The listing builds one solid part. Answer for the finished solid, in the listing's coordinates (mm). A direction names the side the tool comes from. Give positions to 0.01 mm unless a question says otherwise; leave off trailing zeros. Write each loop counter-clockwise with the first axis right and the second up, starting at its lowest first coordinate (ties: lowest second). Pieces come first, ordered by that corner, then holes. Notation, with made-up numbers: M -1.5,15.5 L 25.5,15.5 A23 ccw 25.5,41.5 Z; hole C 75,60.25 d8. An arc over 180 degrees is marked long. Return JSON: item names as keys, results as strings.
from build123d import *

# Parameters (mm, degrees)
F0_W     = 110
F0_H     = 40
F1_DEPTH = 2
F2_W     = 45
F2_H     = 29
F3_DEPTH = 2.001
F4_R     = 2
F5_R     = 4


with BuildPart() as f1:
    # F0 (on Top) → F1 (new body)
    with BuildSketch(Plane.XY):
        Rectangle(F0_W, F0_H)
    extrude(amount=F1_DEPTH)

    # F2 (on face) → F3 (cut, through all)
    with BuildSketch(Plane.XY.offset(2)):
        Rectangle(F2_W, F2_H)
    extrude(amount=-F3_DEPTH, mode=Mode.SUBTRACT)

    # F4
    f4_edges = [f1.edges().sort_by_distance(p)[0] for p in [
        (-22.5, 14.5, 1),
        (22.5, 14.5, 1),
        (-22.5, -14.5, 1),
        (22.5, -14.5, 1),
    ]]
    fillet(f4_edges, radius=F4_R)

    # F5
    f5_edges = [f1.edges().sort_by_distance(p)[0] for p in [
        (-55, -20, 1),
        (-55, 20, 1),
        (55, 20, 1),
        (55, -20, 1),
    ]]
    fillet(f5_edges, radius=F5_R)


solid = f1.part
Item 1: Determine the mould class of faces 3 (the flat face through (55, 0, 1)), 4 (the cylindrical face through (53.797, -18.859, 1.014)), 5 (the cylindrical face through (-21.9, -13.93, 0.99)) for opening direction Y: +Y half, -Y half, draft (parallel to the pull), parting line (faces both ways), or undercut.
Geometry results:
{"face 3": "draft", "face 4": "-Y half", "face 5": "undercut"}
Item 2: A cutting plane is placed at A-A, the plane y = 9. Write down the section's boundary in (x, z).
Geometry results:
{"outline": "M -55,0 L -22.5,0 L -22.5,2 L -55,2 Z; M 22.5,0 L 55,0 L 55,2 L 22.5,2 Z"}
Item 3: Find the intervals of material crossed by line 1 (Y direction, x = 2.5, z = 0.4); line 2 (X direction, y = -2, z = 1.8); line 3 (X direction, y = 13.5, z = 1.25), in increasing order.
Geometry results:
{"line 1": "y = -20 to -14.5, 14.5 to 20", "line 2": "x = -55 to -22.5, 22.5 to 55", "line 3": "x = -55 to -22.23, 22.23 to 55"}
Item 4: A cutting plane is placed at C-C, the plane z = 0.8. Write down the section's boundary in (x, y), plus the area to 3 significant figures.
Geometry results:
{"outline": "M -55,-16 A4 ccw -51,-20 L 51,-20 A4 ccw 55,-16 L 55,16 A4 ccw 51,20 L -51,20 A4 ccw -55,16 Z; hole M -22.5,-12.5 A2 ccw -20.5,-14.5 L 20.5,-14.5 A2 ccw 22.5,-12.5 L 22.5,12.5 A2 ccw 20.5,14.5 L -20.5,14.5 A2 ccw -22.5,12.5 Z", "area": "3,080 mm2"}
Item 5: Which of the six approach directions +Z, -Z, +X, -X, +Y, -Y give full straight-line access (tool end or side, diameter ignored) to faces 1 (the cylindrical face through (-21.9, 13.93, 0.99)), 2 (the flat face through (-1, 18, 2))?
Geometry results:
{"face 1": "+Z, -Z", "face 2": "+Z, +X, -X, +Y, -Y"}
Item 6: A cutting plane is placed at B-B, the plane x = -15. Write down the section's boundary in (y, z), plus the area to 3 significant figures.
Geometry results:
{"outline": "M -20,0 L -14.5,0 L -14.5,2 L -20,2 Z; M 14.5,0 L 20,0 L 20,2 L 14.5,2 Z", "area": "22.0 mm2"}
